Part model, mm, in its own coordinate system. A direction names the side the tool comes from. Round coordinates to 2 decimals unless told otherwise and drop trailing zeros. Order: outer loops, then holes, each group sorted by start corner. A loop starts at its lowest first (then second) coordinate and runs counter-clockwise, first axis right, second up. Notation, with made-up numbers: (71, 71) - (124, 71) arc R17 ccw to (124, 104) - close; hole circle Ø11 at (0, 69). An arc over 180 degrees is marked (long way). Return JSON: item names as keys, results as strings. Group by question number.
Item 1: Probe probe 1 along Z at (x, y) = (-3.25, -3.75) (3 decimals); probe 2 along Z at (x, y) = (-2.75, -1.25) (3 decimals); probe 3 along Y at (x, z) = (0, 42). List the from-to ranges inside material, lowest first.
Item 2: Two-plate mould, pull along Z, no slides. Class faces 3 (the face through (-2.9, 0.6, 55.1)), 4 (the face through (0, 0, 58.175)), 5 (the face through (0, 0, 0)), 6 (the face through (-1.38, -6.2, 2.07)): released by +Z, released by -Z, zero draft, split by the parting line, or undercut.
Item 3: Saw through at C-C on z = 16. List the corners of the cut face in (x, y), and give its area (3 significant figures).
Item 4: Tool access for faces 1 (the face through (-3, 0, 53.175)), 2 (the face through (-3.42, 3.13, 57.11)): list every direction of +Z, -Z, +X, -X, +Y, -Y with a clear straight run to the whole face (end or side of a thin tool).
Item 5: Drop flat-ended pins along their axis: pin 1 (6 mm diameter, centred on y = -2.5, z = 19.5, fed in from +X); pin 2 (1.5 mm diameter, centred on y = -4.5, z = 22.5, fed in from +X); pin 3 (6 mm diameter, centred on y = -4, z = 50.5, fed in from -X). Give the stop position or say it passes through.
```python
from build123d import *

# Parameters (mm, degrees)
F0_R     = 6.35
F1_DEPTH = 3.175
F2_R     = 4.6355
F3_DEPTH = 55
F6_SIZE  = 1


# Not quite as in the source:
# - a length typed as a fraction of an inch, garbled in the dataset ("3 / 203.2 mm" for 3/8 in), is restored


with BuildPart() as f1:
    # F0 (on Top) → F1 (new body)
    with BuildSketch(Plane.XY):
        Circle(F0_R)
    extrude(amount=F1_DEPTH)

    # F2 (on face) → F3 (join)
    with BuildSketch(Plane.XY.offset(3.175)):
        Circle(F2_R)
    extrude(amount=F3_DEPTH)

    # F4 (on Right) → F5 (revolve, cut)
    with BuildSketch(Plane.YZ):
        Polygon((-2.8230392858, 55.0202994616), (-4.8230392858, 56.175), (-4.8230392858, 53.175), (-2.8230392858, 53.175), align=None)
    revolve(axis=Axis((0, 0, 58.175), (0, 0, 1)), mode=Mode.SUBTRACT)

    # F6
    f6_edges = [f1.edges().sort_by_distance(p)[0] for p in [
        (-6.35, 0, 0),
    ]]
    chamfer(f6_edges, length=F6_SIZE)


solid = f1.part
```
Filled in:
{
 "1": {"probe 1": "z = 0 to 3.175", "probe 2": "z = 0 to 53.175, 55.134 to 58.175", "probe 3": "y = -4.64 to 4.64"},
 "2": {"face 3": "undercut", "face 4": "released by +Z", "face 5": "released by -Z", "face 6": "zero draft"},
 "3": {"outline": "circle Ø9.27 at (0, 0)", "area": "67.5 mm^2"},
 "4": {"face 1": "none", "face 2": "+Z"},
 "5": {"pin 1": "stops at x = 4.64", "pin 2": "stops at x = 2.72", "pin 3": "stops at x = -4.53"}
}
